The model under review builds one solid part; all positions refer to its coordinate system, in mm. Round coordinates to 2 decimals unless told otherwise and drop trailing zeros. Loops run counter-clockwise (first coordinate to the right, second up) from the corner with the lowest first, then second, coordinate; pieces in that order, holes last. Notation, with made-up numbers: M 17.5,20.5 L 27.5,20.5 A21 ccw 27.5,32.5 Z; hole C 24,-20 d8. An arc over 180 degrees is marked long. Answer as a JSON object with one key per item and string values. Group by question number.
Item 1: Consider section D-D (y = -35.5). Give the boundary of the cut face in (x, z), and give its area (3 significant figures).
Item 2: To check wall thickness, follow line 1 (Y direction, x = 1, z = -0.25); line 2 (Z direction, x = 0.25, y = -36); line 3 (Y direction, x = 4.75, z = -9). State the ranges of each line that lie inside material, in increasing order.
Item 3: Consider section A-A (x = 0). Give the boundary of the cut face in (y, z).
Item 4: Consider section C-C (x = 5.5). Give the boundary of the cut face in (y, z).
Item 5: Insertion check: P1, Ø2, axis at y = -24, z = -8, coming from the -X side; P2, Ø5, axis at y = -31, z = -5, coming from the +X side; P3, Ø6, axis at x = -8, y = -10, coming from the +Z side. Each pin has a flat end and moves straight along its axis. Give the tip position at first contact, or say it passes through.
Item 6: The part is to be moulded in two halves that separate along Y. For faces 1 (the face through (0, 10.25, -1)), 2 (the face through (3, 0, 0)), 3 (the face through (-14.985, -19.72, 0.66)), 4 (the face through (0, 5, -1)), say which applies: +Y half, -Y half, draft (parallel to the pull), parting line (faces both ways), or undercut.
Item 7: Consider section B-B (z = 3.5). Give the boundary of the cut face in (x, y), and give its area (3 significant figures).
```python
from build123d import *

# Parameters (mm, degrees)
F0_R     = 15
F1_DEPTH = 40
F2_R     = 1
F3_DEPTH = 10
F7_W     = 1.6538074706
F7_H     = 5.6983865798
F8_DEPTH = 0.25


# Not quite as in the source:
# - the program builds the solid bodies; features that only make, move or delete a surface that nothing else refers to are left out


with BuildPart() as f1:
    # F0 (on Front) → F1 (new body)
    with BuildSketch(Plane.XZ):
        Circle(F0_R)
    extrude(amount=F1_DEPTH)

    # F2 (on face) → F3 (join)
    with BuildSketch(Plane(origin=(0, 0, 0), x_dir=(-1, 0, 0), z_dir=(0, 1, 0))):
        Circle(F2_R)
    extrude(amount=F3_DEPTH)

    # F7 (on face) → F8 (join)
    with BuildSketch(Plane(origin=(0, 10, 0), x_dir=(-1, 0, 0), z_dir=(0, 1, 0))):
        with BuildLine():
            Line((2.032, -12.968), (6.6767431337, 0))
            ThreePointArc((6.6767431337, 0), (0, 6.6767431337), (-6.6767431337, 0))
            Line((-6.6767431337, 0), (-2.032, -12.968))
            Line((-2.032, -12.968), (2.032, -12.968))
        make_face()
        with Locations((0, -9.3933474272)):
            Rectangle(F7_W, F7_H, mode=Mode.SUBTRACT)
    extrude(amount=F8_DEPTH)


solid = f1.part
```
Geometry results:
{
 "1": {"outline": "C 0,0 d30", "area": "707 mm^2"},
 "2": {"line 1": "y = -40 to 0, 10 to 10.25", "line 2": "z = -15 to 15", "line 3": "y = -40 to 0"},
 "3": {"outline": "M -40,-15 L 0,-15 L 0,-1 L 10,-1 L 10,-6.54 L 10.25,-6.54 L 10.25,6.68 L 10,6.68 L 10,1 L 0,1 L 0,15 L -40,15 Z; M 10,-12.97 L 10.25,-12.97 L 10.25,-12.24 L 10,-12.24 Z"},
 "4": {"outline": "M -40,-13.96 L 0,-13.96 L 0,13.96 L -40,13.96 Z; M 10,-3.29 L 10.25,-3.29 L 10.25,3.79 L 10,3.79 Z"},
 "5": {"P1": "stops at x = -13.27", "P2": "stops at x = 14.79", "P3": "stops at z = 14.14"},
 "6": {"face 1": "+Y half", "face 2": "undercut", "face 3": "draft", "face 4": "undercut"},
 "7": {"outline": "M -14.59,-40 L 14.59,-40 L 14.59,0 L -14.59,0 Z; M -5.69,10 L 5.69,10 L 5.69,10.25 L -5.69,10.25 Z", "area": "1,170 mm^2"}
}
